Check sheet for the modelled part. Datum: model origin and axes. Units: mm. A direction names the side the tool comes from. Give positions to 0.01 mm unless a question says otherwise; leave off trailing zeros. Loops run counter-clockwise (first coordinate to the right, second up) from the corner with the lowest first, then second, coordinate; pieces in that order, holes last. Notation, with made-up numbers: M -36,50 L -10,50 A23 ccw -10,67 Z; hole C -0.5,-11.75 d11. An arc over 180 degrees is marked long. Use one line per item in the form item = value.
from build123d import *

# Parameters (mm, degrees)
ESQUISSE1_W             = 45
ESQUISSE1_H             = 24
ESQUISSE1_R             = 4
BOSS_EXTRU_1_DEPTH      = 25
ESQUISSE2_W             = 15
ESQUISSE2_H             = 13
ESQUISSE2_R             = 2.5
BOSS_EXTRU_2_DEPTH      = 20
ESQUISSE3_R             = 1.75
ENL_V_MAT_EXTRU_1_DEPTH = 20


with BuildPart() as part:
    # Esquisse1 → Boss.-Extru.1 (new body)
    with BuildSketch(Plane.XY):
        with Locations((4.197614073, -0.216957606)):
            Rectangle(ESQUISSE1_W, ESQUISSE1_H)
        with Locations((-8.302385927, -0.216957606)):
            Circle(ESQUISSE1_R, mode=Mode.SUBTRACT)
        with Locations((16.697614073, -0.216957606)):
            Circle(ESQUISSE1_R, mode=Mode.SUBTRACT)
    extrude(amount=BOSS_EXTRU_1_DEPTH)

    # Esquisse2 → Boss.-Extru.2 (add)
    with BuildSketch(Plane.XY.offset(25)):
        with Locations((4.197614073, -18.716957606)):
            Rectangle(ESQUISSE2_W, ESQUISSE2_H)
        with Locations((4.197614073, -18.216957606)):
            Circle(ESQUISSE2_R, mode=Mode.SUBTRACT)
    extrude(amount=-BOSS_EXTRU_2_DEPTH)

    # Esquisse3 → Enlèv. mat.-Extru.1 (cut)
    with BuildSketch(Plane.ZY.offset(3.302385927)):
        with Locations((20, -22.716957606)):
            Circle(ESQUISSE3_R)
    extrude(amount=-ENL_V_MAT_EXTRU_1_DEPTH, mode=Mode.SUBTRACT)


solid = part.part
1) Section check C-C (y = 2.5). Record the cut outline in (x, z).
Evaluation:
outline = M -18.3,0 L -11.24,0 L -11.24,25 L -18.3,25 Z; M -5.37,0 L 13.76,0 L 13.76,25 L -5.37,25 Z; M 19.63,0 L 26.7,0 L 26.7,25 L 19.63,25 Z
2) Set-up check for faces 1 (the face through (11.698, -19, 15)), 2 (the face through (-3.302, -19, 15)), 3 (the face through (2, -20, 5)): record each of +Z, -Z, +X, -X, +Y, -Y from which the full face is reachable in a straight line by a thin tool's end or side.
Evaluation:
face_1 = +Z, -Z, +X, -Y
face_2 = +Z, -Z, -X, -Y
face_3 = -Z, +X, -X, -Y
3) Section check D-D (z = 11.5). Record the cut outline in (x, y).
Evaluation:
outline = M -18.3,-12.22 L -3.3,-12.22 L -3.3,-25.22 L 11.7,-25.22 L 11.7,-12.22 L 26.7,-12.22 L 26.7,11.78 L -18.3,11.78 Z; hole C -8.3,-0.22 d8; hole C 4.2,-18.22 d5; hole C 16.7,-0.22 d8
4) Section check A-A (z = 19.25). Record the cut outline in (x, y).
Evaluation:
outline = M -18.3,-12.22 L -3.3,-12.22 L -3.3,-21.14 L 11.7,-21.14 L 11.7,-12.22 L 26.7,-12.22 L 26.7,11.78 L -18.3,11.78 Z; M -3.3,-25.22 L 11.7,-25.22 L 11.7,-24.3 L -3.3,-24.3 Z; hole C -8.3,-0.22 d8; hole C 4.2,-18.22 d5; hole C 16.7,-0.22 d8
5) Scan lines: line 1 (X direction, y = -18, z = 15.25); line 2 (Y direction, x = 4, z = 20); line 3 (X direction, y = -1, z = 6.25) (3 decimals). Record each from-to range of solid material in increasing order.
Evaluation:
line_1 = -3.3 to 1.71, 6.69 to 11.7
line_2 = -25.22 to -24.47, -20.97 to -20.71, -15.72 to 11.78
line_3 = -18.302 to -12.225, -4.38 to 12.775, 20.62 to 26.698
6) Section check B-B (x = 3). Record the cut outline in (y, z).
Evaluation:
outline = M -25.22,5 L -20.41,5 L -20.41,25 L -25.22,25 Z; M -16.02,5 L -12.22,5 L -12.22,0 L 11.78,0 L 11.78,25 L -16.02,25 Z; hole C -22.72,20 d3.5
7) Release check for a two-part mould opening along Z. For faces 4 (the face through (4, -2, 25)), 5 (the face through (26.698, 0, 12)), 6 (the face through (4.093, -21.534, 18.71)) record: pulls with the +Z half, pulls with the -Z half, needs draft (parallel to the pull), parting line crosses it, or undercut.
Evaluation:
face_4 = pulls with the +Z half
face_5 = needs draft
face_6 = undercut
8) Depth check by flat-ended pin: pin 1 Ø8 at (x, y) = (4.2, -18.22) entering from -Z; pin 2 Ø4.5 at (y, z) = (-22.72, 20) entering from +X; pin 3 Ø5 at (x, y) = (-8.3, -0.22) entering from -Z (3 decimals); pin 4 Ø10 at (x, z) = (19.5, 6.5) entering from -Y. Enter the tip coordinate at first touch or a pass-through.
Evaluation:
pin_1 = 5
pin_2 = 11.7
pin_3 = through
pin_4 = -12.22
